```python
from build123d import *

# Parameters (mm, degrees)
EXTRUDE_1_DEPTH          = 90
EXTRUDE_1_DEPTH_BACK     = 250
SKETCH_1_R               = 10
CUT_EXTRUDE_1_DEPTH      = 251.399680511
CUT_EXTRUDE_1_DEPTH_BACK = 251.399680511
SKETCH_2_R               = 2.5
CHAMFER_1_SIZE           = 1
CUT_EXTRUDE_START        = -58
SKETCH_3_OUTSIDE_W       = 90.234
SKETCH_3_OUTSIDE_H       = 90.234
SKETCH_3_OUTSIDE_R       = 9.5
CUT_EXTRUDE_2_DEPTH      = 1.3
SKETCH_4_OUTSIDE_W       = 90.234
SKETCH_4_OUTSIDE_H       = 90.234
SKETCH_4_OUTSIDE_R       = 8.5
CUT_EXTRUDE_3_DEPTH      = 28
HOLE_WIZARD_M3_1_D       = 2.5
HOLE_WIZARD_M3_1_DEPTH   = 16.748924226
HOLE_WIZARD_M3_1_TIP     = 0.751075774
SKETCH_12_OUTSIDE_W      = 90.234
SKETCH_12_OUTSIDE_H      = 90.234
SKETCH_12_OUTSIDE_R      = 9
CUT_EXTRUDE_4_DEPTH      = 33
EXTRUDE_2_DEPTH          = 33
PATTERN_CIRCULAR_1_COUNT = 6
SKETCH_14_OUTSIDE_W      = 91.326
SKETCH_14_OUTSIDE_H      = 92.272
SKETCH_14_OUTSIDE_R      = 9
CUT_EXTRUDE_5_DEPTH      = 2
EXTRUDE_START            = 25
SKETCH_15_R              = 9
EXTRUDE_3_DEPTH          = 25
CUT_EXTRUDE_START_2      = -25
SKETCH_16_OUTSIDE_W      = 96.308
SKETCH_16_OUTSIDE_H      = 97.254
SKETCH_16_OUTSIDE_R      = 8.5
CUT_EXTRUDE_6_DEPTH      = 1


# Read off the part's stored shape, not the designer's step: M18 机械螺纹 螺柱1
with BuildPart() as part:
    # 草图1 → 凸台-拉伸1 (new, two sides: drawn at the far end of the back side and taken through both)
    with BuildSketch(Plane(origin=(0, 0, 0), x_dir=(1, 0, 0), z_dir=(0, 1, 0)).offset(-EXTRUDE_1_DEPTH_BACK)):
        with Locations(Location((0, 0, 0), (0, 0, 90))):
            Circle(SKETCH_1_R)
    extrude(amount=EXTRUDE_1_DEPTH + EXTRUDE_1_DEPTH_BACK)

    # 草图2 → 切除-拉伸1 (cut, two sides: drawn at the far end of the back side and taken through both)
    with BuildSketch(Plane(origin=(0, 0, 0), x_dir=(0, 0, -1), z_dir=(1, 0, 0)).offset(-CUT_EXTRUDE_1_DEPTH_BACK)):
        Circle(SKETCH_2_R)
    extrude(amount=CUT_EXTRUDE_1_DEPTH + CUT_EXTRUDE_1_DEPTH_BACK, mode=Mode.SUBTRACT)

    # 倒角1
    chamfer_1_edges = [part.edges().sort_by_distance(p)[0] for p in [
        (0, 90, 10),
    ]]
    chamfer(chamfer_1_edges, length=CHAMFER_1_SIZE)

    # 草图3 outside → 切除-拉伸2 (cut)
    with BuildSketch(Plane(origin=(0, 0, 0), x_dir=(1, 0, 0), z_dir=(0, 1, 0)).offset(CUT_EXTRUDE_START)):
        Rectangle(SKETCH_3_OUTSIDE_W, SKETCH_3_OUTSIDE_H)
        with Locations(Location((0, 0, 0), (0, 0, 270))):
            Circle(SKETCH_3_OUTSIDE_R, mode=Mode.SUBTRACT)
    extrude(amount=CUT_EXTRUDE_2_DEPTH, mode=Mode.SUBTRACT)

    # 草图4 outside → 切除-拉伸3 (cut)
    with BuildSketch(Plane(origin=(0, 90, 0), x_dir=(1, 0, 0), z_dir=(0, 1, 0))):
        Rectangle(SKETCH_4_OUTSIDE_W, SKETCH_4_OUTSIDE_H)
        with Locations(Location((0, 0, 0), (0, 0, 270))):
            Circle(SKETCH_4_OUTSIDE_R, mode=Mode.SUBTRACT)
    extrude(amount=-CUT_EXTRUDE_3_DEPTH, mode=Mode.SUBTRACT)

    # M3 螺纹孔1
    with Locations(Plane(origin=(0, 90, 0), x_dir=(1, 0, 0), z_dir=(0, 1, 0))):
        with Locations((4, 0), (-4, 0)):
            Hole(HOLE_WIZARD_M3_1_D / 2, depth=HOLE_WIZARD_M3_1_DEPTH)
            with Locations((0, 0, -(HOLE_WIZARD_M3_1_DEPTH + HOLE_WIZARD_M3_1_TIP / 2))):  # 118° drill point
                Cone(0, HOLE_WIZARD_M3_1_D / 2, HOLE_WIZARD_M3_1_TIP, mode=Mode.SUBTRACT)

    # 草图12 outside → 切除-拉伸4 (cut)
    with BuildSketch(Plane.XZ.offset(250)):
        Rectangle(SKETCH_12_OUTSIDE_W, SKETCH_12_OUTSIDE_H)
        with Locations(Location((0, 0, 0), (0, 0, 270))):
            Circle(SKETCH_12_OUTSIDE_R, mode=Mode.SUBTRACT)
    extrude(amount=-CUT_EXTRUDE_4_DEPTH, mode=Mode.SUBTRACT)

    # 草图13 → 凸台-拉伸2 (add)
    with BuildSketch(Plane.XZ.offset(250)):
        with BuildLine():
            Line((-2.5, -10.712142643), (-2.5, 10.712142643))
            ThreePointArc((-2.5, 10.712142643), (0, 11), (2.5, 10.712142643))
            Line((2.5, 10.712142643), (2.5, -10.712142643))
            ThreePointArc((2.5, -10.712142643), (0, -11), (-2.5, -10.712142643))
        make_face()
    extrude_2 = extrude(amount=-EXTRUDE_2_DEPTH)

    # 阵列(圆周)1: 凸台-拉伸2 ×6 about axis
    pattern_circular_1_axis = Axis((0, 0, 0), (0, 1, 0))
    for i in range(1, PATTERN_CIRCULAR_1_COUNT):
        add(extrude_2.rotate(pattern_circular_1_axis, i * 360 / PATTERN_CIRCULAR_1_COUNT))

    # 草图14 outside → 切除-拉伸5 (cut)
    with BuildSketch(Plane.XZ.offset(217)):
        Rectangle(SKETCH_14_OUTSIDE_W, SKETCH_14_OUTSIDE_H)
        with Locations(Location((0, 0, 0), (0, 0, 270))):
            Circle(SKETCH_14_OUTSIDE_R, mode=Mode.SUBTRACT)
    extrude(amount=-CUT_EXTRUDE_5_DEPTH, mode=Mode.SUBTRACT)

    # 草图15 → 凸台-拉伸3 (add)
    with BuildSketch(Plane.XZ.offset(250).offset(EXTRUDE_START)):
        with Locations(Location((0, 0, 0), (0, 0, 270))):
            Circle(SKETCH_15_R)
    extrude(amount=-EXTRUDE_3_DEPTH)

    # 草图16 outside → 切除-拉伸6 (cut)
    with BuildSketch(Plane.XZ.offset(275).offset(CUT_EXTRUDE_START_2)):
        Rectangle(SKETCH_16_OUTSIDE_W, SKETCH_16_OUTSIDE_H)
        with Locations(Location((0, 0, 0), (0, 0, 90))):
            Circle(SKETCH_16_OUTSIDE_R, mode=Mode.SUBTRACT)
    extrude(amount=CUT_EXTRUDE_6_DEPTH, mode=Mode.SUBTRACT)

    # M18 机械螺纹 螺柱1 outline → M18 机械螺纹 螺柱1 (revolve, cut)
    with BuildSketch(Plane.XY):
        Polygon((9, -273.647), (7.647, -275), (9, -275), align=None)
    revolve(axis=Axis((0, 0, 0), (0, 1, 0)), mode=Mode.SUBTRACT)


solid = part.part
```
Design review of the part built by this model. Coordinates are the model's own, in mm. A direction names the side the tool comes from. Coordinates: 2 decimals unless noted, no trailing zeros. Order: outer loops, then holes, each group sorted by start corner. A loop starts at its lowest first (then second) coordinate and runs counter-clockwise, first axis right, second up. Notation, with made-up numbers: M 72.25,-19 L 99.25,-19 A19 ccw 99.25,-4 Z; hole C 68.5,75.25 d5. An arc over 180 degrees is marked long. Answer as a JSON object with one key per item and string values. Group by question number.
1) Tool access review of faces 1 (the cylindrical face through (2.703, -262.482, -8.584)), 2 (the flat face through (0, 90, 0)), 3 (the cylindrical face through (-5.78, -57.36, -7.54)), 4 (the cylindrical face through (9.76, 1.82, 2.17)): name each direction out of +Z, -Z, +X, -X, +Y, -Y from which nothing blocks a thin tool from reaching the whole face with its end or side.
2) Wall thickness on L1, parallel to Y at x = -9.25, z = -3.5; L2, parallel to Z at x = -4, y = 81.25; L3, parallel to Z at x = -5, y = 46: over which ranges is each line inside the solid? List them lowest first.
3) For pin 1 (6 mm diameter, centred on y = 0, z = 0, fed in from -X); pin 2 (1.9 mm diameter, centred on x = 1, z = -10, fed in from +Y); pin 3 (12 mm diameter, centred on x = 3, y = -198, fed in from -Z), all flat-tipped, find the tip position at first contact; note any pin that passes through.
4) Add section A-A, the plane y = -223.5. Write out the cut boundary in (x, z).
5) Add section B-B, the plane y = -158.5. Write out the cut boundary in (x, z).
6) Mouldability with a two-part tool opening along Y and no side actions: class faces 5 (the flat face through (0, -275, 0)), 6 (the cylindrical face through (9.76, -137.6, 2.17)), 7 (the flat face through (9, -56.7, 4)) as pulls with the +Y half, pulls with the -Y half, needs draft (parallel to the pull), parting line crosses it, or undercut.
Computed values:
{
 "1": {"face 1": "-Y", "face 2": "+Z, -Z, +X, -X, +Y", "face 3": "none", "face 4": "+Y"},
 "2": {"L1": "y = -250 to -217, -215 to -58, -56.7 to 62", "L2": "z = -7.5 to -1.25, 1.25 to 7.5", "L3": "z = -8.66 to 8.66"},
 "3": {"pin 1": "stops at x = -10", "pin 2": "stops at y = 62", "pin 3": "stops at z = -10"},
 "4": {"outline": "M -10.53,-3.19 A11 ccw -8.03,-7.52 L -6.24,-6.49 A9 ccw -2.5,-8.65 L -2.5,-10.71 A11 ccw 2.5,-10.71 L 2.5,-8.65 A9 ccw 6.24,-6.49 L 8.03,-7.52 A11 ccw 10.53,-3.19 L 8.74,-2.16 A9 ccw 8.74,2.16 L 10.53,3.19 A11 ccw 8.03,7.52 L 6.24,6.49 A9 ccw 2.5,8.65 L 2.5,10.71 A11 ccw -2.5,10.71 L -2.5,8.65 A9 ccw -6.24,6.49 L -8.03,7.52 A11 ccw -10.53,3.19 L -8.74,2.16 A9 ccw -8.74,-2.16 Z"},
 "5": {"outline": "C 0,0 d20"},
 "6": {"face 5": "pulls with the -Y half", "face 6": "needs draft", "face 7": "undercut"}
}
